Autodesk Inventor part; units mm, degrees
ref_plane "YZ Plane" through (0, 0, 0) normal (1, 0, 0) x (0, 1, 0)
ref_plane "XZ Plane" through (0, 0, 0) normal (0, 1, 0) x (-1, 0, 0)
ref_plane "XY Plane" through (0, 0, 0) normal (0, 0, 1) x (1, 0, 0)
sketch "Sketch1" plane through (0, 0, 0) normal (0, 0, 1) x (1, 0, 0)
  line L0 (-9.5, -9.5) -> (9.5, -9.5)
  line L1 (9.5, -9.5) -> (9.5, 9.5)
  line L2 (9.5, 9.5) -> (-9.5, 9.5)
  line L3 (-9.5, 9.5) -> (-9.5, -9.5)
  line L4 (-9.5, -9.5) -> (9.5, 9.5) construction
  line L5 (9.5, -9.5) -> (-9.5, 9.5) construction
  point P0 (0, 0)
  dimension "d0" = 19
  dimension "d1" = 19
extrude "Extrusion1" add sketch "Sketch1" along normal blind 8
sketch "Sketch2" plane through (0, 0, 8) normal (0, 0, 1) x (1, 0, 0)
  line L0 (-9.5, 1.6684) -> (-1.6676, 1.6684)
  line L1 (1.7162, 1.6684) -> (9.5, 1.6684)
  line L2 (-1.7, -9.5) -> (-1.7, -1.7316)
  line L3 (-1.6676, 1.6684) -> (-1.6676, 9.5)
  line L4 (1.7, -9.5) -> (1.7, -1.7316)
  line L5 (1.7162, 1.6684) -> (1.7162, 9.5)
  line L6 (-9.5, -1.7316) -> (-1.7, -1.7316)
  line L7 (1.7, -1.7316) -> (9.5, -1.7316)
  line L8 (-9.5, 1.6684) -> (-9.5, -1.7316)
  line L9 (-1.7, -9.5) -> (1.7, -9.5)
  line L10 (9.5, -1.7316) -> (9.5, 1.6684)
  line L11 (-1.6676, 9.5) -> (1.7162, 9.5)
  point P0 (0, 0)
extrude "Extrusion2" add sketch "Sketch2" along normal blind 2
properties part number "Stop Block"
Build history of the part. All positions in model axes, mm. A direction names the side the tool comes from. Round coordinates to 2 decimals unless told otherwise and drop trailing zeros. Loops run counter-clockwise (first coordinate to the right, second up) from the corner with the lowest first, then second, coordinate; pieces in that order, holes last. Notation, with made-up numbers: (61, 55) -> (94, 55) arc R13 cw to (94, 78) -> close; hole circle Ø6 at (37, 32). An arc over 180 degrees is marked (long way). One line per item, written item: value. Start each with the question number.
Q1. Cut at A-A on y = 6.75. List the corners of the cut face in (x, z).
Q2. Probe line 1 along Z through (x, y) = (-3.25, 8.75); line 2 along Y through (x, z) = (2.75, 8.5); line 3 along X through (y, z) = (5.5, 8.25). List the from-to ranges inside material, lowest first.
Q3. Cut at B-B on z = 9.5. List the corners of the cut face in (x, y), plus the area to 3 significant figures.
Q4. 3-axis set-ups, long thin cutter, end or side, ignore diameter. For faces 1 (the face through (-1.668, 6, 9)), 2 (the face through (1.716, 6, 9)), 3 (the face through (-6, -1.732, 9)), 4 (the face through (-1, 0, 10)), 5 (the face through (6, -6, 8)): which of +Z, -Z, +X, -X, +Y, -Y reach the whole face in a straight line?
Q5. Drop flat-ended pins along their axis: pin 1 Ø1 at (y, z) = (-4, 9.5) entering from +X; pin 2 Ø1 at (y, z) = (-5, 9) entering from -X; pin 3 Ø8 at (x, y) = (-5, 4) entering from -Z; pin 4 Ø4 at (x, y) = (-6.5, 6.5) entering from +Z. Give the stop position or say it passes through.
Q6. Cut at C-C on x = -2.75. List the corners of the cut face in (y, z).
Computed:
1. outline: (-9.5, 0) -> (9.5, 0) -> (9.5, 8) -> (1.72, 8) -> (1.72, 10) -> (-1.67, 10) -> (-1.67, 8) -> (-9.5, 8) -> close
2. line 1: 0 to 8
2. line 2: -1.73 to 1.67
2. line 3: -1.67 to 1.72
3. outline: (-9.5, -1.73) -> (-1.7, -1.73) -> (-1.7, -9.5) -> (1.7, -9.5) -> (1.7, -1.73) -> (9.5, -1.73) -> (9.5, 1.67) -> (1.72, 1.67) -> (1.72, 9.5) -> (-1.67, 9.5) -> (-1.67, 1.67) -> (-9.5, 1.67) -> close
3. area: 118 mm²
4. face 1: +Z, -X, +Y
4. face 2: +Z, +X, +Y
4. face 3: +Z, -X, -Y
4. face 4: +Z, +X, -X, +Y, -Y
4. face 5: +Z, +X, -Y
5. pin 1: x = 1.7
5. pin 2: x = -1.7
5. pin 3: z = 0
5. pin 4: z = 8
6. outline: (-9.5, 0) -> (9.5, 0) -> (9.5, 8) -> (1.67, 8) -> (1.67, 10) -> (-1.73, 10) -> (-1.73, 8) -> (-9.5, 8) -> close
